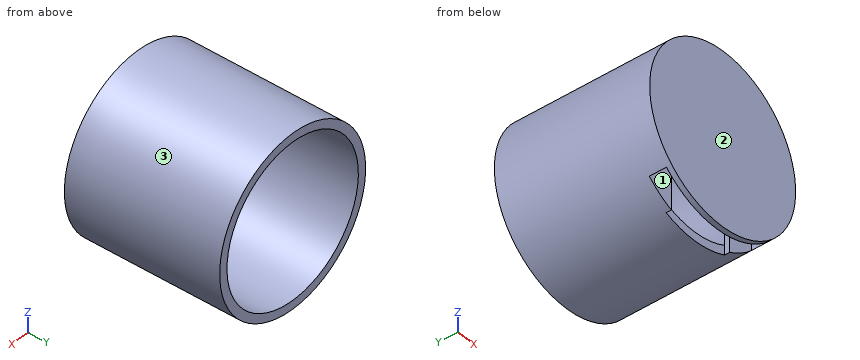
from build123d import *

# Parameters (mm, degrees)
SKETCH1_R           = 50
BOSS_EXTRUDE1_DEPTH = 13
SKETCH2_W           = 70
SKETCH2_H           = 55
CUT_EXTRUDE1_DEPTH  = 10
CUT_EXTRUDE3_START  = -10
CUT_EXTRUDE3_DEPTH  = 10
SKETCH6_R           = 50
BOSS_EXTRUDE5_DEPTH = 3
SKETCH11_W          = 40
SKETCH11_H          = 65
CUT_EXTRUDE12_DEPTH = 10
CUT_EXTRUDE13_START = -10
CUT_EXTRUDE13_DEPTH = 10
SKETCH13_R          = 50
BOSS_EXTRUDE6_DEPTH = 75
SKETCH14_R          = 45
CUT_EXTRUDE14_DEPTH = 75


with BuildPart() as part:
    # Sketch1 → Boss-Extrude1 (new body)
    with BuildSketch(Plane(origin=(0, 0, 0), x_dir=(1, 0, 0), z_dir=(0, 1, 0))):
        with Locations(Location((0, 0, 0), (0, 0, 90))):
            Circle(SKETCH1_R)
    extrude(amount=BOSS_EXTRUDE1_DEPTH)

    # Sketch2 → Cut-Extrude1 (cut)
    with BuildSketch(Plane(origin=(0, 13, 0), x_dir=(1, 0, 0), z_dir=(0, 1, 0))):
        with Locations((-0.015145616, 8.297810168)):
            Rectangle(SKETCH2_W, SKETCH2_H)
    extrude(amount=-CUT_EXTRUDE1_DEPTH, mode=Mode.SUBTRACT)

    # Sketch3 → Cut-Extrude3 (cut)
    with BuildSketch(Plane(origin=(0, 13, 0), x_dir=(1, 0, 0), z_dir=(0, 1, 0)).offset(CUT_EXTRUDE3_START)):
        with BuildLine():
            Line((-35.015145616, 35.692290169), (34.984854384, 35.72198152))
            ThreePointArc((34.984854384, 35.72198152), (-0.021208106, 49.999995502), (-35.015145616, 35.692290169))
        make_face()
    extrude(amount=CUT_EXTRUDE3_DEPTH, mode=Mode.SUBTRACT)

    # Sketch6 → Boss-Extrude5 (add)
    with BuildSketch(Plane(origin=(0, 13, 0), x_dir=(1, 0, 0), z_dir=(0, 1, 0))):
        with Locations(Location((0, 0, 0), (0, 0, 270))):
            Circle(SKETCH6_R)
    extrude(amount=BOSS_EXTRUDE5_DEPTH)

    # Sketch11 → Cut-Extrude12 (cut)
    with BuildSketch(Plane(origin=(0, 16, 0), x_dir=(1, 0, 0), z_dir=(0, 1, 0))):
        with Locations((0, 13.32575695)):
            Rectangle(SKETCH11_W, SKETCH11_H)
    extrude(amount=-CUT_EXTRUDE12_DEPTH, mode=Mode.SUBTRACT)

    # Sketch12 → Cut-Extrude13 (cut)
    with BuildSketch(Plane(origin=(0, 16, 0), x_dir=(1, 0, 0), z_dir=(0, 1, 0)).offset(CUT_EXTRUDE13_START)):
        with BuildLine():
            Line((-20, 45.82575695), (20, 45.82575695))
            ThreePointArc((20, 45.82575695), (0, 50), (-20, 45.82575695))
        make_face()
    extrude(amount=CUT_EXTRUDE13_DEPTH, mode=Mode.SUBTRACT)

    # Sketch13 → Boss-Extrude6 (add)
    with BuildSketch(Plane(origin=(0, 16, 0), x_dir=(1, 0, 0), z_dir=(0, 1, 0))):
        with Locations(Location((0, 0, 0), (0, 0, 270))):
            Circle(SKETCH13_R)
    extrude(amount=BOSS_EXTRUDE6_DEPTH)

    # Sketch14 → Cut-Extrude14 (cut)
    with BuildSketch(Plane(origin=(0, 91, 0), x_dir=(1, 0, 0), z_dir=(0, 1, 0))):
        with Locations(Location((0, 0, 0), (0, 0, 270))):
            Circle(SKETCH14_R)
    extrude(amount=-CUT_EXTRUDE14_DEPTH, mode=Mode.SUBTRACT)


solid = part.part
Geometry check sheet. Reference: the model listing, model coordinates, mm. Face numbers are marked on the shaded views. Give positions to 0.01 mm unless a question says otherwise; leave off trailing zeros. Order: outer loops, then holes, each group sorted by start corner. A loop starts at its lowest first (then second) coordinate and runs counter-clockwise, first axis right, second up. Notation, with made-up numbers: (-40, -35.75) - (12, -35.75) arc R25 ccw to (12, -2.75) - close; hole circle Ø9 at (26, -32). An arc over 180 degrees is marked (long way). Answer as a JSON object with one key per item and string values.
(1) Cross-section at D-D (x = -37). Record the cut outline in (y, z), then the cut area to 3 significant figures.
Report:
{"outline": "(0, -33.63) - (91, -33.63) - (91, -25.61) - (16, -25.61) - (16, 25.61) - (91, 25.61) - (91, 33.63) - (0, 33.63) - close", "area": "2,280 mm^2"}
(2) Depth check by flat-ended pin: pin 1 Ø8 at (y, z) = (8, -13) entering from +X; pin 2 Ø3 at (x, y) = (-10.5, 8.5) entering from -Z; pin 3 Ø10 at (x, z) = (-39, 4) entering from +Y. Enter the tip coordinate at first touch or a pass-through.
Report:
{"pin 1": "x = 49.18", "pin 2": "z = 19.2", "pin 3": "y = 16"}
(3) Draft check along X on the marked faces 1, 2 and 3. Enter one of: released by +X, released by -X, zero draft, split by the parting line, or undercut.
Report:
{"face 1": "undercut", "face 2": "zero draft", "face 3": "split by the parting line"}
(4) Cross-section at C-C (z = 0). Record the cut outline in (x, y), then the cut area to 3 significant figures.
Report:
{"outline": "(-50, 0) - (50, 0) - (50, 91) - (45, 91) - (45, 16) - (20, 16) - (20, 13) - (34.98, 13) - (34.98, 3) - (-35.02, 3) - (-35.02, 13) - (-20, 13) - (-20, 16) - (-45, 16) - (-45, 91) - (-50, 91) - close", "area": "1,530 mm^2"}
(5) Material ranges on line 1 (Y direction, x = 22, z = -0.5); line 2 (Z direction, x = 0, y = 47.5), recorded low to high.
Report:
{"line 1": "0 to 3, 13 to 16", "line 2": "-50 to -45, 45 to 50"}
(6) Cross-section at B-B (y = 83.5). Record the cut outline in (x, z), then the cut area to 3 significant figures.
Report:
{"outline": "circle Ø100 at (0, 0); hole circle Ø90 at (0, 0)", "area": "1,490 mm^2"}
